Verification items for the finished model (mm, model axes). A direction names the side the tool comes from. Coordinates: 2 decimals unless noted, no trailing zeros. Order: outer loops, then holes, each group sorted by start corner. A loop starts at its lowest first (then second) coordinate and runs counter-clockwise, first axis right, second up. Notation, with made-up numbers: M 20,14.25 L 71,14.25 A21 cw 71,44.25 Z; hole C 25,87 d10. An arc over 180 degrees is marked long. Return JSON: item names as keys, results as strings.
```python
from build123d import *

# Parameters (mm, degrees)
SKETCH1_W            = 15.875
SKETCH1_H            = 15.875
BOSS_EXTRUDE1_DEPTH  = 9.525
SKETCH2_R            = 2.38125
BOSS_EXTRUDE2_DEPTH  = 1.5875
LPATTERN1_COUNT      = 2
LPATTERN1_PITCH      = 7.9375
LPATTERN1_COUNT_DIR2 = 2
LPATTERN1_PITCH_DIR2 = 7.9375
SHELL1_T             = -1.5875
SKETCH3_R            = 3.175
SKETCH3_R_2          = 2.38125
BOSS_EXTRUDE9_DEPTH  = 7.9375


with BuildPart() as part:
    # Sketch1 → Boss-Extrude1 (new body)
    with BuildSketch(Plane.XY):
        with Locations((7.9375, 7.9375)):
            Rectangle(SKETCH1_W, SKETCH1_H)
    extrude(amount=BOSS_EXTRUDE1_DEPTH)

    # Sketch2 → Boss-Extrude2 (add)
    with BuildSketch(Plane.XY.offset(9.525)):
        with Locations((3.96875, 11.90625)):
            Circle(SKETCH2_R)
    boss_extrude2 = extrude(amount=BOSS_EXTRUDE2_DEPTH)

    # LPattern1: Boss-Extrude2 2 × 2
    with Locations(*[(j * LPATTERN1_PITCH_DIR2, -i * LPATTERN1_PITCH, 0) for i in range(LPATTERN1_COUNT) for j in range(LPATTERN1_COUNT_DIR2) if (i, j) != (0, 0)]):
        add(boss_extrude2)

    # Shell1
    shell1_openings = [part.faces().sort_by_distance(p)[0] for p in [
        (7.9375, 7.9375, 0),
    ]]
    offset(amount=SHELL1_T, openings=shell1_openings, kind=Kind.INTERSECTION)

    # Sketch3 → Boss-Extrude9 (add)
    with BuildSketch(Plane(origin=(0, 0, 7.9375), x_dir=(-1, 0, 0), z_dir=(0, 0, -1))):
        with Locations((-7.9375, 7.9375)):
            Circle(SKETCH3_R)
        with Locations((-7.9375, 7.9375)):
            Circle(SKETCH3_R_2, mode=Mode.SUBTRACT)
    extrude(amount=BOSS_EXTRUDE9_DEPTH)


solid = part.part
```
Q1. Go/stop test with flat-tipped pins: pin 1 (1.8 mm diameter, centred on x = 11.91, y = 3.97, fed in from -Z); pin 2 (1.3 mm diameter, centred on x = 12, y = 4, fed in from -Z) (3 decimals). Record where each tip stops, or that it passes through.
Values:
{"pin 1": "z = 7.94", "pin 2": "z = 9.525"}
Q2. Cross-section at C-C, the plane x = 13.75. Record the boundary of the cut face in (y, z) (1 decimal), and give its area (3 significant figures).
Values:
{"outline": "M 0,0 L 1.6,0 L 1.6,7.9 L 14.3,7.9 L 14.3,0 L 15.9,0 L 15.9,9.5 L 13.4,9.5 L 13.4,11.1 L 10.4,11.1 L 10.4,9.5 L 5.5,9.5 L 5.5,11.1 L 2.5,11.1 L 2.5,9.5 L 0,9.5 Z", "area": "60.0 mm^2"}
Q3. Draft check along X on faces 4 (the face through (0, 8, 5)), 5 (the face through (8, 0, 5)), 6 (the face through (8, 14.288, 4)). Enter one of: pulls with the +X half, pulls with the -X half, needs draft (parallel to the pull), parting line crosses it, or undercut.
Values:
{"face 4": "pulls with the -X half", "face 5": "needs draft", "face 6": "undercut"}
Q4. Cross-section at D-D, the plane y = 2.5. Record the boundary of the cut face in (x, z) (1 decimal).
Values:
{"outline": "M 0,0 L 1.6,0 L 1.6,7.9 L 14.3,7.9 L 14.3,0 L 15.9,0 L 15.9,9.5 L 13.8,9.5 L 13.8,11.1 L 10,11.1 L 10,9.5 L 5.8,9.5 L 5.8,11.1 L 2.1,11.1 L 2.1,9.5 L 0,9.5 Z"}
Q5. Cross-section at B-B, the plane z = 9. Record the boundary of the cut face in (x, y) (1 decimal), and give its area (3 significant figures).
Values:
{"outline": "M 0,0 L 15.9,0 L 15.9,15.9 L 0,15.9 Z; hole C 4,4 d1.6; hole C 4,11.9 d1.6; hole C 11.9,4 d1.6; hole C 11.9,11.9 d1.6", "area": "244 mm^2"}
Q6. Tool access check on faces 1 (the face through (4, 4, 9.525)), 2 (the face through (8, 15.875, 5)), 3 (the face through (11.39, 9.58, 10.31)). Record the directions out of +Z, -Z, +X, -X, +Y, -Y that give a thin tool (end or side, any length) a straight path to the whole face; none if there is none.
Values:
{"face 1": "-Z", "face 2": "+Z, -Z, +X, -X, +Y", "face 3": "+Z"}
Q7. Material ranges on line 1 along Y through (x, z) = (12, 8.5) (3 decimals); line 2 along X through (y, z) = (12.75, 1.5) (1 decimal), recorded low to high.
Values:
{"line 1": "0 to 3.181, 4.757 to 11.118, 12.694 to 15.875", "line 2": "0 to 1.6, 14.3 to 15.9"}
Q8. Cross-section at A-A, the plane z = 6.5. State how many separate pieces and enclosed holes the cut face has, and give its area (3 significant figures).
Values:
{"separate pieces": "2", "enclosed holes": "2", "area": "105 mm^2"}
